Autodesk Inventor part; units mm, degrees
ref_plane "Work Plane1" through (0, 0, 19.5) normal (0, 0, 1) x (1, 0, 0)
ref_plane "YZ Plane" through (0, 0, 0) normal (1, 0, 0) x (0, 1, 0)
ref_plane "XZ Plane" through (0, 0, 0) normal (0, 1, 0) x (-1, 0, 0)
sketch "Sketch1" plane through (0, 0, 0) normal (0, 0, 1) x (1, 0, 0)
  line L0 (0, 0) -> (0, 3.4207)
  line L1 (0, 0) -> (9.2929, 0)
  line L2 (21.15, -21.15) -> (-21.15, -21.15)
  line L3 (-21.15, -21.15) -> (-21.15, 21.15)
  line L4 (-21.15, 21.15) -> (21.15, 21.15)
  line L5 (21.15, 21.15) -> (21.15, -21.15)
  point P0 (0, 21.15)
  point P1 (21.15, 0)
  dimension "d0" = 42.3
  dimension "d1" = 42.3
extrude "Extrusion1" add sketch "Sketch1" along normal blind 39
sketch "Sketch2" plane through (0, 0, 0) normal (0, 0, -1) x (-1, 0, 0)
  line L0 (-21.15, 21.15) -> (-21.15, -21.15)
  circle A0 centre (-15.5, 15.5) radius 2
  circle A1 centre (15.5, 15.5) radius 2
  line L1 (-15.5, 15.5) -> (15.5, 15.5)
  line L2 (0, 0) -> (0, 5.3355)
  line L3 (0, 0) -> (5.467, 0)
  circle A2 centre (-15.5, -15.5) radius 2
  circle A3 centre (15.5, -15.5) radius 2
  line L4 (-15.5, -15.5) -> (15.5, -15.5)
  line L5 (-21.15, 21.15) -> (-11.15, 21.15)
  line L6 (-11.15, 21.15) -> (-11.15, 11.15)
  line L7 (-11.15, 11.15) -> (-21.15, 11.15)
  line L8 (-21.15, 11.15) -> (-21.15, 21.15)
  line L9 (21.15, 21.15) -> (11.15, 21.15)
  line L10 (11.15, 21.15) -> (11.15, 11.15)
  line L11 (11.15, 11.15) -> (21.15, 11.15)
  line L12 (21.15, 11.15) -> (21.15, 21.15)
  line L13 (21.15, -21.15) -> (11.15, -21.15)
  line L14 (11.15, -21.15) -> (11.15, -11.15)
  line L15 (11.15, -11.15) -> (21.15, -11.15)
  line L16 (21.15, -11.15) -> (21.15, -21.15)
  line L17 (-21.15, -21.15) -> (-11.15, -21.15)
  line L18 (-11.15, -21.15) -> (-11.15, -11.15)
  line L19 (-11.15, -11.15) -> (-21.15, -11.15)
  line L20 (-21.15, -11.15) -> (-21.15, -21.15)
  circle A4 centre (0, 0) radius 11
  point P0 (0, 15.5)
  point P1 (0, -15.5)
  dimension "d4" = 4
  dimension "d5" = 4
  dimension "d6" = 31
  dimension "d7" = 31
  dimension "d8" = 10
  dimension "d9" = 10
  dimension "d10" = 10
  dimension "d11" = 10
  dimension "d12" = 10
  dimension "d13" = 10
  dimension "d14" = 10
  dimension "d15" = 10
  dimension "d20" = 22
extrude "Extrusion2" add sketch "Sketch2" along normal blind 1 contours A0 | L5 L6 L7 L0 | A1 | L10 L9 L12 L11 | A3 | L14 L15 L16 L13 | A2 | L19 L18 L17 L0
extrude "Extrusion3" cut sketch "Sketch2" along normal mid plane 2 contours A0 | A1 | A3 | A2
extrude "Extrusion4" add sketch "Sketch2" along normal blind 1 contours A4
fillet "Fillet1" radius 3 4 edges at (11.15, 11.15, -0.5) (11.15, -11.15, -0.5) (-11.15, -11.15, -0.5) (-11.15, 11.15, -0.5)
chamfer "Chamfer1" distance 2 angle 45 4 edges at (21.15, -21.15, 19) (-21.15, -21.15, 19) (-21.15, 21.15, 19) (21.15, 21.15, 19)
sketch "Sketch3" plane through (0, 0, -1) normal (0, 0, -1) x (-1, 0, 0)
  circle A0 centre (0, 0) radius 11
  circle A1 centre (0, 0) radius 2.5
  dimension "d27" = 5
extrude "Extrusion5" add sketch "Sketch3" along normal blind 22 contours A1
ref_plane "Work Plane1" through (0, 0, 19.5) normal (0, 0, 1) x (1, 0, 0)
mirror "Mirror1" about plane through (0, 0, 19.5) normal (0, 0, 1) of "Extrusion3"
sketch "Sketch4" plane through (21.15, -11.15, 0) normal (1, 0, 0) x (0, 0, -1)
  line L0 (-39, -8) -> (-39, 30.3)
  line L1 (-35, 14.15) -> (-33, 14.15)
  line L2 (-33, 14.15) -> (-33, 8.15)
  line L3 (-33, 8.15) -> (-35, 8.15)
  line L4 (-35, 8.15) -> (-35, 14.15)
  line L5 (-39, 11.15) -> (-36.6866, 11.15)
  point P0 (0, 11.15)
  point P1 (-35, 11.15)
  dimension "d31" = 2
  dimension "d32" = 6
  dimension "d33" = 4
extrude "Extrusion6" add sketch "Sketch4" along normal blind 4
sketch "Sketch6" plane through (0, 0, 19.5) normal (0, 0, 1) x (1, 0, 0)
  line L0 (-21.15, 19.15) -> (-19.15, 21.15)
  line L1 (-19.15, 21.15) -> (19.15, 21.15)
  line L2 (19.15, 21.15) -> (21.15, 19.15)
  line L3 (21.15, 19.15) -> (21.15, -19.15)
  line L4 (21.15, -19.15) -> (19.15, -21.15)
  line L5 (19.15, -21.15) -> (-19.15, -21.15)
  line L6 (-19.15, -21.15) -> (-21.15, -19.15)
  line L7 (-21.15, -19.15) -> (-21.15, 19.15)
  line L8 (-17.7379, 17.7408) -> (-17.7408, 17.7379)
  line L9 (-17.7408, -17.7379) -> (-17.7379, -17.7408)
  line L10 (17.7379, -17.7408) -> (17.7408, -17.7379)
  line L11 (17.7408, 17.7379) -> (17.7379, 17.7408)
  line L12 (-21.15, 14.9074) -> (-14.9074, 21.15)
  line L13 (-18.0287, 18.0287) -> (18.0287, 18.0287)
  line L14 (18.0287, 18.0287) -> (18.0287, -18.0287)
  line L15 (18.0287, -18.0287) -> (-18.0287, -18.0287)
  line L16 (-18.0287, -18.0287) -> (-18.0287, 18.0287)
  line L17 (-21.15, 14.9074) -> (-21.15, 19.15)
  line L18 (-19.15, 21.15) -> (-21.15, 19.15)
  line L19 (-19.15, 21.15) -> (-14.9074, 21.15)
  line L20 (-14.9074, -21.15) -> (-21.15, -14.9074)
  line L21 (-14.9074, -21.15) -> (-19.15, -21.15)
  line L22 (-21.15, -19.15) -> (-19.15, -21.15)
  line L23 (-21.15, -19.15) -> (-21.15, -14.9074)
  line L24 (21.15, -14.9074) -> (14.9074, -21.15)
  line L25 (21.15, -14.9074) -> (21.15, -19.15)
  line L26 (19.15, -21.15) -> (21.15, -19.15)
  line L27 (19.15, -21.15) -> (14.9074, -21.15)
  line L28 (14.9074, 21.15) -> (21.15, 14.9074)
  line L29 (14.9074, 21.15) -> (19.15, 21.15)
  line L30 (21.15, 19.15) -> (19.15, 21.15)
  line L31 (21.15, 19.15) -> (21.15, 14.9074)
  line L32 (-21.15, 14.9074) -> (-21.15, -14.9074)
  line L33 (-14.9074, -21.15) -> (14.9074, -21.15)
  line L34 (21.15, -14.9074) -> (21.15, 14.9074)
  line L35 (14.9074, 21.15) -> (-14.9074, 21.15)
  point P0 (0, 0)
  point P1 (18.0287, -18.0287)
  dimension "d43" = 3
  dimension "d46" = 360
extrude "Extrusion8" cut sketch "Sketch6" along normal mid plane 26 contours L0 L1 L12 L7 | L12 L16 L20 L7 | L1 L28 L13 L12 | L20 L5 L6 L7 | L1 L2 L3 L28 | L15 L24 L5 L20 | L28 L3 L24 L14 | L24 L3 L4 L5
properties part number "Stepper Motor NEMA 17" material "Rubber"
CAD build for the part. Positions are in the model's coordinates, mm. A direction names the side the tool comes from. Coordinates: 2 decimals unless noted, no trailing zeros. Order: outer loops, then holes, each group sorted by start corner. A loop starts at its lowest first (then second) coordinate and runs counter-clockwise, first axis right, second up. Notation, with made-up numbers: M 40,-28 L 53,-28 A19 ccw 53,6 Z; hole C -17,-20.75 d1. An arc over 180 degrees is marked long. Write each question's results on one line, items separated by ' | '. Start each with the question number.
Q1. Cut at A-A (y = 0). List the corners of the cut face in (x, z), then the cut area to 3 significant figures.
Q2. Flat gauge pins, fed straight in: P1, Ø3, axis at x = 23, y = -1, coming from the +Z side; P2, Ø1.5, axis at y = -2.5, z = -6.5, coming from the +X side; P3, Ø7, axis at y = 8.5, z = 34.5, coming from the +X side. Where does each tip first touch, or does it go through?
Q3. Cut at B-B (x = 0). List the corners of the cut face in (y, z), then the cut area to 3 significant figures.
Q4. Drill centre lines: probe 1 along Y at (x, z) = (-15.5, 38.7); probe 2 along Z at (x, y) = (-10.5, 18.5); probe 3 along X at (y, z) = (17, 27). Where is each one in solid material? Low to high. Write a range as from..to.
Q5. Pull direction Y, two halves, no side cores. Call faces 1 (the flat face through (-20.1, 20.2, 35.7)), 2 (the flat face through (15, 16, 38)), 3 (the flat face through (21.15, 0, 3)), 4 (the cylindrical face through (15.76, -17.483, 0.014)): +Y half, -Y half, draft (parallel to the pull), parting line (faces both ways), or undercut.
Q6. Cut at D-D (z = -14). List the corners of the cut face in (x, y), then the cut area to 3 significant figures.
Q7. Which spindle directions (+Z, -Z, +X, -X, +Y, -Y) get a long thin tool onto all of the face, cutting with end or side? Do faces 5 (the cylindrical face through (12.01, -12.05, -0.51)), 6 (the flat face through (23, 0, 33)), 7 (the cylindrical face through (-15.24, 13.517, 38.507)). Say none if no direction does.
Found:
1) outline: M -21.15,0 L -11,0 L -11,-1 L -2.5,-1 L -2.5,-23 L 2.5,-23 L 2.5,-1 L 11,-1 L 11,0 L 21.15,0 L 21.15,6.5 L 18.03,6.5 L 18.03,32.5 L 21.15,32.5 L 21.15,33 L 25.15,33 L 25.15,35 L 21.15,35 L 21.15,39 L -21.15,39 L -21.15,32.5 L -18.03,32.5 L -18.03,6.5 L -21.15,6.5 Z | area: 1,630 mm²
2) P1: z = 35 | P2: x = 1.79 | P3: x = 21.15
3) outline: M -21.15,0 L -11,0 L -11,-1 L -2.5,-1 L -2.5,-23 L 2.5,-23 L 2.5,-1 L 11,-1 L 11,0 L 21.15,0 L 21.15,6.5 L 18.03,6.5 L 18.03,32.5 L 21.15,32.5 L 21.15,39 L -21.15,39 L -21.15,32.5 L -18.03,32.5 L -18.03,6.5 L -21.15,6.5 Z | area: 1,620 mm²
4) probe 1: -21.15..-17.5, -13.5..13.5, 17.5..21.15 | probe 2: 0..6.5, 32.5..39 | probe 3: -18.03..18.03
5) face 1: +Y half | face 2: undercut | face 3: draft | face 4: undercut
6) outline: C 0,0 d5 | area: 19.6 mm²
7) face 5: -Z | face 6: -Z, +X, +Y, -Y | face 7: +Z
